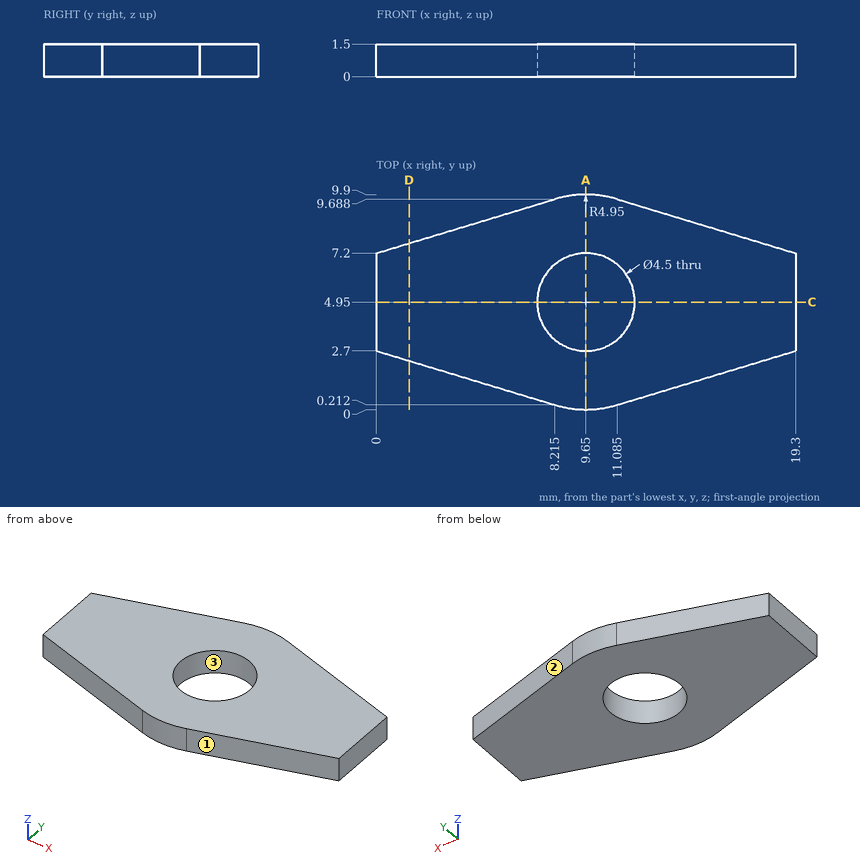
Source: three-view drawing plus pictorial views. Frame: mm from the lowest corner of the part. Give positions to 0.01 mm unless a question says otherwise; leave off trailing zeros. Order: outer loops, then holes, each group sorted by start corner. A loop starts at its lowest first (then second) coordinate and runs counter-clockwise, first axis right, second up. Notation, with made-up numbers: (80.25, 42) -> (121.25, 42) arc R28 cw to (121.25, 77) -> close; hole circle Ø11 at (42.25, 59). An arc over 180 degrees is marked (long way). Write each question's results on one line, items separated by ' | '. Start each with the question number.
Item 1: Line query: line 1 (Y direction, x = 9.65, z = 0.85); line 2 (X direction, y = 3.5, z = 0.9); line 3 (X direction, y = 4.25, z = 0.4). Output: solid intervals per line, ascending.
Item 2: Mould query, pull axis Y, two halves, no side actions, for the marked faces 1, 2 and 3. Classes: pulls with the +Y half, pulls with the -Y half, needs draft (parallel to the pull), parting line crosses it, or undercut.
Item 3: Cut plane D-D on x = 1.5. Return the cut outline in (y, z) (1 decimal).
Item 4: Cut plane A-A on x = 9.65. Return the cut outline in (y, z).
Item 5: Contact query for flat-ended pins moving along their axis: P1, Ø1, axis at x = 8.5, y = 2, coming from the -Z side; P2, Ø3.5, axis at x = 9.65, y = 4.95, coming from the +Z side (3 decimals). Output: stop coordinate, or through.
Item 6: Cut plane C-C on y = 4.95. Return the cut outline in (x, z), then the cut area to 3 significant figures.
Established:
1) line 1: 0 to 2.7, 7.2 to 9.9 | line 2: 0 to 7.93, 11.37 to 19.3 | line 3: 0 to 7.51, 11.79 to 19.3
2) face 1: pulls with the -Y half | face 2: pulls with the +Y half | face 3: undercut
3) outline: (2.2, 0) -> (7.7, 0) -> (7.7, 1.5) -> (2.2, 1.5) -> close
4) outline: (0, 0) -> (2.7, 0) -> (2.7, 1.5) -> (0, 1.5) -> close; (7.2, 0) -> (9.9, 0) -> (9.9, 1.5) -> (7.2, 1.5) -> close
5) P1: z = 0 | P2: through
6) outline: (0, 0) -> (7.4, 0) -> (7.4, 1.5) -> (0, 1.5) -> close; (11.9, 0) -> (19.3, 0) -> (19.3, 1.5) -> (11.9, 1.5) -> close | area: 22.2 mm^2
